Geometry check sheet. Reference: drawing and pictorial views, mm from the part's lowest x, y, z. A direction names the side the tool comes from. Coordinates: 2 decimals unless noted, no trailing zeros. Loops run counter-clockwise (first coordinate to the right, second up) from the corner with the lowest first, then second, coordinate; pieces in that order, holes last. Notation, with made-up numbers: (18, 89.25) - (35, 89.25) arc R27 ccw to (35, 114.25) - close; hole circle Ø9 at (15.5, 59.5). An arc over 180 degrees is marked (long way). One line per item, written item: value.
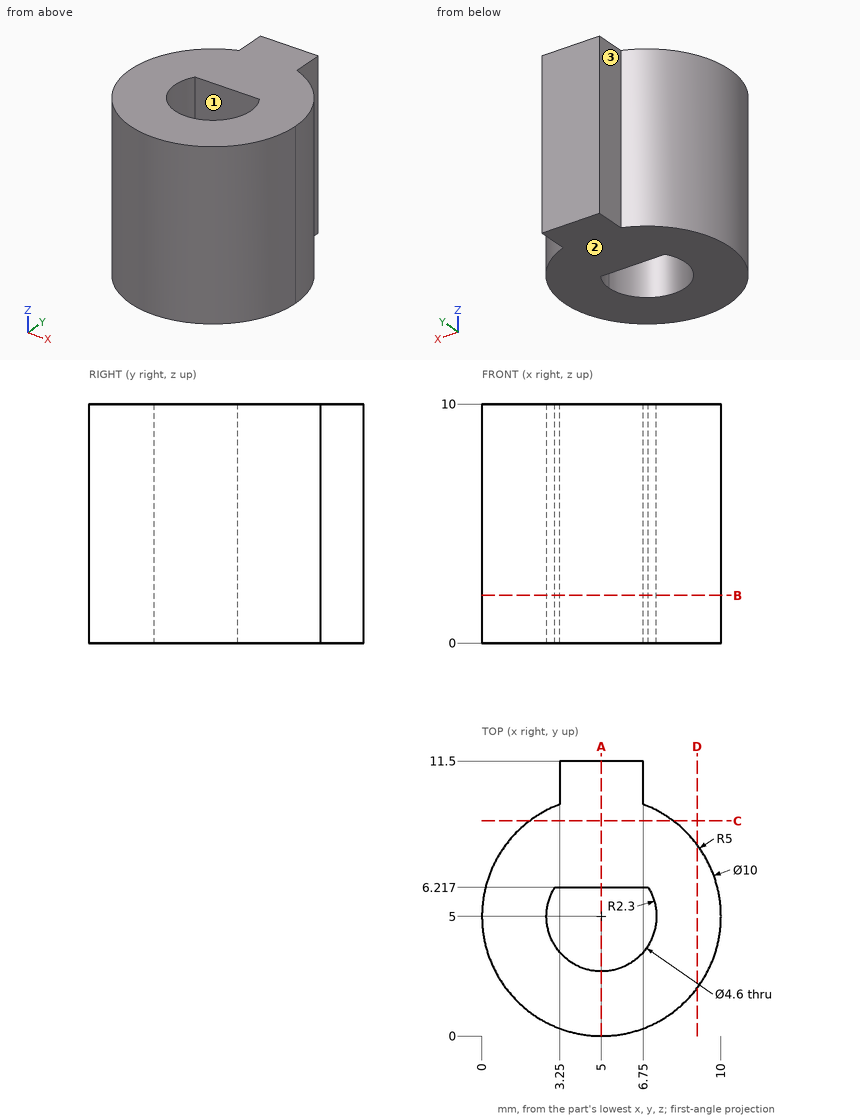
(1) Cross-section at C-C on y = 9. Record the cut outline in (x, z).
Reply:
outline: (2, 0) - (8, 0) - (8, 10) - (2, 10) - close
(2) Access from +Z, -Z, +X, -X, +Y, -Y to the whole of each face (thin tool, end or side, straight path). Record for the marked faces 1, 2 and 3.
Reply:
face 1: +Z, -Z
face 2: -Z, +X, -X, +Y, -Y
face 3: +Z, -Z, -X, +Y
(3) Material ranges on probe 1 along Y at (x, z) = (5, 3.5); probe 2 along X at (y, z) = (5, 5.5); probe 3 along Y at (x, z) = (6, 1) (1 decimal), recorded low to high. Write a range as from..to.
Reply:
probe 1: 0..2.7, 6.22..11.5
probe 2: 0..2.7, 7.3..10
probe 3: 0.1..2.9, 6.2..11.5
(4) Cross-section at A-A on x = 5. Record the cut outline in (y, z).
Reply:
outline: (0, 0) - (2.7, 0) - (2.7, 10) - (0, 10) - close; (6.22, 0) - (11.5, 0) - (11.5, 10) - (6.22, 10) - close
(5) Cross-section at B-B on z = 2. Record the cut outline in (x, y).
Reply:
outline: (3.25, 9.68) arc R5 ccw (long way) to (6.75, 9.68) - (6.75, 11.5) - (3.25, 11.5) - close; hole (3.05, 6.22) arc R2.3 ccw (long way) to (6.95, 6.22) - close
(6) Go/stop test with flat-tipped pins: pin 1 Ø6 at (x, z) = (7.5, 9) entering from +Y; pin 2 Ø0.9 at (y, z) = (10.5, 5.5) entering from -X; pin 3 Ø1.5 at (x, z) = (7.5, 9) entering from -Y; pin 4 Ø1.5 at (y, z) = (10, 5) entering from +X (1 decimal). Record where each tip stops, or that it passes through.
Reply:
pin 1: y = 11.5
pin 2: x = 3.25
pin 3: y = 0.32
pin 4: x = 7.6
